For this review, take the finished solid that the model builds, in its own axes (mm). Face numbers are marked on the shaded views. Round coordinates to 2 decimals unless told otherwise and drop trailing zeros. Order: outer loops, then holes, each group sorted by start corner. A loop starts at its lowest first (then second) coordinate and runs counter-clockwise, first axis right, second up. Notation, with made-up numbers: M -18.75,-24 L 14.25,-24 A17 cw 14.25,-17 Z; hole C -4.5,72.5 d11. An arc over 180 degrees is marked long. Put each result on its own line as item: value.
from build123d import *

# Parameters (mm, degrees)
SKETCH1_R           = 22.5
SKETCH1_R_2         = 2.25
SKETCH1_R_3         = 12.5
BOSS_EXTRUDE1_DEPTH = 20
CHAMFER1_SIZE       = 1


with BuildPart() as part:
    # Sketch1 → Boss-Extrude1 (new body)
    with BuildSketch(Plane(origin=(0, 0, 0), x_dir=(1, 0, 0), z_dir=(0, 1, 0))):
        with Locations(Location((0, 0, 0), (0, 0, 270))):
            Circle(SKETCH1_R)
        with Locations(Location((-17.5, 0, 0), (0, 0, 270))):
            Circle(SKETCH1_R_2, mode=Mode.SUBTRACT)
        with Locations(Location((0, 17.5, 0), (0, 0, 270))):
            Circle(SKETCH1_R_2, mode=Mode.SUBTRACT)
        with Locations(Location((17.5, 0, 0), (0, 0, 270))):
            Circle(SKETCH1_R_2, mode=Mode.SUBTRACT)
        with Locations(Location((0, -17.5, 0), (0, 0, 270))):
            Circle(SKETCH1_R_2, mode=Mode.SUBTRACT)
        with Locations(Location((0, 0, 0), (0, 0, 270))):
            Circle(SKETCH1_R_3, mode=Mode.SUBTRACT)
    extrude(amount=BOSS_EXTRUDE1_DEPTH)

    # Chamfer1
    chamfer1_edges = [part.edges().sort_by_distance(p)[0] for p in [
        (0, 0, -19.75),
        (0, 20, -19.75),
        (17.5, 0, -2.25),
        (17.5, 20, -2.25),
        (0, 0, -22.5),
        (0, 0, 15.25),
        (0, 20, 15.25),
        (0, 20, -22.5),
        (-17.5, 0, -2.25),
        (-17.5, 20, -2.25),
        (0, 0, -12.5),
        (0, 20, -12.5),
    ]]
    chamfer(chamfer1_edges, length=CHAMFER1_SIZE)


solid = part.part
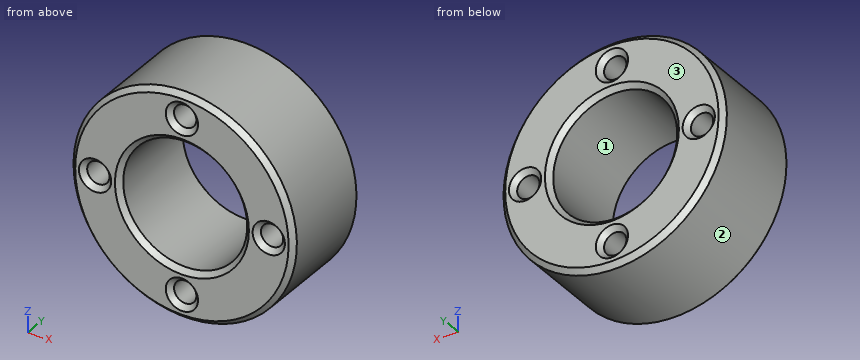
(1) Add section B-B on y = 6.5. Give the boundary of the cut face in (x, z).
A:
outline: C 0,0 d45; hole C -17.5,0 d4.5; hole C 0,0 d25; hole C 0,-17.5 d4.5; hole C 0,17.5 d4.5; hole C 17.5,0 d4.5
(2) To check wall thickness, follow L1, parallel to X at y = 11, z = 0; L2, parallel to Z at x = -1.5, y = 4.5; L3, parallel to Z at x = 1, y = 1.25. State the ranges of each line that lie inside material, in increasing order.
A:
L1: x = -22.5 to -19.75, -15.25 to -12.5, 12.5 to 15.25, 19.75 to 22.5
L2: z = -22.45 to -19.18, -15.82 to -12.41, 12.41 to 15.82, 19.18 to 22.45
L3: z = -22.48 to -19.52, -15.48 to -12.46, 12.46 to 15.48, 19.52 to 22.48
(3) Insertion check: pin 1 Ø2 at (x, z) = (17.5, 15.5) entering from -Y; pin 2 Ø6 at (x, z) = (17.5, 0) entering from +Y; pin 3 Ø3.5 at (x, z) = (0, -17.5) entering from +Y; pin 4 Ø2 at (x, y) = (-15, 17.5) entering from +Z. Each pin has a flat end and moves straight along its axis. Give the tip position at first contact, or say it passes through.
A:
pin 1: stops at y = 0.88
pin 2: stops at y = 19.75
pin 3: passes through
pin 4: stops at z = 17.61
(4) Add section A-A on x = 0. State how many separate pieces and enclosed holes the cut face has, then the cut area to 3 significant figures.
A:
separate pieces: 4
enclosed holes: 0
area: 212 mm2
(5) Draft analysis for pull direction X (two halves, no side actions). For the marked faces 1, 2 and 3, state which applies: released by +X, released by -X, zero draft, split by the parting line, or undercut.
A:
face 1: undercut
face 2: split by the parting line
face 3: zero draft
